from build123d import *

# Parameters (mm, degrees)
SKETCH2_R             = 0.5
BASE_DEPTH            = 2
M3_CLEARANCE_HOLE1_D  = 3.4
M4X0_7_TAPPED_HOLE1_D = 3.3


with BuildPart() as part:
    # Sketch2 → Base (new body, symmetric)
    with BuildSketch(Plane.XY):
        with BuildLine():
            Line((-18.5, 0), (18.5, 0))
            ThreePointArc((18.5, 0), (19.560660172, 0.439339828), (20, 1.5))
            Line((20, 1.5), (20, 1.8041591))
            ThreePointArc((20, 1.8041591), (20.327112072, 2.739217337), (21.165778543, 3.266450459))
            Line((21.165778543, 3.266450459), (46.691257218, 9.100556377))
            ThreePointArc((46.691257218, 9.100556377), (49.699443623, 13.891257218), (44.908742782, 16.899443623))
            Line((44.908742782, 16.899443623), (12.649834838, 9.526344449))
            ThreePointArc((12.649834838, 9.526344449), (10.989330142, 9.243827753), (9.307620269, 9.149258036))
            Line((9.307620269, 9.149258036), (-9.307620269, 9.149258036))
            ThreePointArc((-9.307620269, 9.149258036), (-10.989330142, 9.243827753), (-12.649834838, 9.526344449))
            Line((-12.649834838, 9.526344449), (-44.908742782, 16.899443623))
            ThreePointArc((-44.908742782, 16.899443623), (-49.699443623, 13.891257218), (-46.691257218, 9.100556377))
            Line((-46.691257218, 9.100556377), (-21.165778543, 3.266450459))
            ThreePointArc((-21.165778543, 3.266450459), (-20.327112072, 2.739217337), (-20, 1.8041591))
            Line((-20, 1.8041591), (-20, 1.5))
            ThreePointArc((-20, 1.5), (-19.560660172, 0.439339828), (-18.5, 0))
        make_face()
        with Locations((-45.8, 13)):
            Circle(SKETCH2_R, mode=Mode.SUBTRACT)
        with Locations((-8, 4)):
            Circle(SKETCH2_R, mode=Mode.SUBTRACT)
        with Locations((8, 4)):
            Circle(SKETCH2_R, mode=Mode.SUBTRACT)
        with Locations((45.8, 13)):
            Circle(SKETCH2_R, mode=Mode.SUBTRACT)
    extrude(amount=BASE_DEPTH, both=True)

    # M3 Clearance Hole1 (through all)
    with Locations(Plane(origin=(0, 4, 2), x_dir=(1, 0, 0), z_dir=(0, 0, 1))):
        with Locations((-8, 0), (8, 0)):
            Hole(M3_CLEARANCE_HOLE1_D / 2)

    # M4x0.7 Tapped Hole1 (through all)
    with Locations(Plane(origin=(0, 0, 2), x_dir=(-1, 0, 0), z_dir=(0, 0, 1))):
        with Locations((-45.8, -13), (45.8, -13)):
            Hole(M4X0_7_TAPPED_HOLE1_D / 2)


solid = part.part
Check sheet for the modelled part. Datum: model origin and axes. Units: mm. A direction names the side the tool comes from. Round coordinates to 2 decimals unless told otherwise and drop trailing zeros. Write each loop counter-clockwise with the first axis right and the second up, starting at its lowest first coordinate (ties: lowest second). Pieces come first, ordered by that corner, then holes. Notation, with made-up numbers: (-37, 67.25) - (-16, 67.25) arc R30 cw to (-16, 104.25) - close; hole circle Ø5 at (18, 69). An arc over 180 degrees is marked (long way). Return JSON: item names as keys, results as strings.
Q1. Draft check along Y on faces 1 (the cylindrical face through (-7.63, 2.34, -0.03)), 2 (the cylindrical face through (49.718, 13.805, 0.028)), 3 (the flat face through (-34.107, 6.224, 0.028)), 4 (the cylindrical face through (47.324, 13.632, -0.028)). Enter one of: released by +Y, released by -Y, zero draft, split by the parting line, or undercut.
Returned:
{"face 1": "undercut", "face 2": "split by the parting line", "face 3": "released by -Y", "face 4": "undercut"}
Q2. Cross-section at D-D (x = 42). Record the boundary of the cut face in (y, z).
Returned:
{"outline": "(8.03, -2) - (16.23, -2) - (16.23, 2) - (8.03, 2) - close"}
Q3. Scan lines: L1, parallel to Y at x = 8, z = 1.15; L2, parallel to X at y = 2.5, z = -1.25; L3, parallel to Y at x = -44.5, z = -1.75. Record each from-to range of solid material in increasing order. Write a range as from..to.
Returned:
{"L1": "y = 0..2.3, 5.7..9.15", "L2": "x = -20.17..-8.8, -7.2..7.2, 8.8..20.17", "L3": "y = 8.6..11.98, 14.02..16.81"}
Q4. Cross-section at A-A (x = -8). Record the boundary of the cut face in (y, z).
Returned:
{"outline": "(0, -2) - (2.3, -2) - (2.3, 2) - (0, 2) - close; (5.7, -2) - (9.15, -2) - (9.15, 2) - (5.7, 2) - close"}
Q5. Cross-section at C-C (z = 0). Record the boundary of the cut face in (x, y), then the cut area to 3 significant figures.
Returned:
{"outline": "(-46.69, 9.1) - (-21.17, 3.27) arc R1.5 cw to (-20, 1.8) - (-20, 1.5) arc R1.5 ccw to (-18.5, 0) - (18.5, 0) arc R1.5 ccw to (20, 1.5) - (20, 1.8) arc R1.5 cw to (21.17, 3.27) - (46.69, 9.1) arc R4 ccw to (44.91, 16.9) - (12.65, 9.53) arc R15 cw to (9.31, 9.15) - (-9.31, 9.15) arc R15 cw to (-12.65, 9.53) - (-44.91, 16.9) arc R4 ccw to start; hole circle Ø3.3 at (-45.8, 13); hole circle Ø3.4 at (-8, 4); hole circle Ø3.4 at (8, 4); hole circle Ø3.3 at (45.8, 13)", "area": "823 mm²"}
Q6. Cross-section at B-B (y = 15.5). Record the boundary of the cut face in (x, z).
Returned:
{"outline": "(-48.92, -2) - (-38.79, -2) - (-38.79, 2) - (-48.92, 2) - close; (38.79, -2) - (48.92, -2) - (48.92, 2) - (38.79, 2) - close"}
Q7. Depth check by flat-ended pin: P1, Ø3, axis at x = -8, y = 4, coming from the -Z side; P2, Ø1.2, axis at x = -2, z = 0.5, coming from the +Y side. Enter the tip coordinate at first touch or a pass-through.
Returned:
{"P1": "passes through", "P2": "stops at y = 9.15"}
Q8. Access from +Z, -Z, +X, -X, +Y, -Y to the whole of each face (thin tool, end or side, straight path). Record for faces 5 (the flat face through (-28.55, 13.16, 0.03)), 6 (the flat face through (-0.7, 8.6, 2)).
Returned:
{"face 5": "+Z, -Z, +Y", "face 6": "+Z, +X, -X, +Y, -Y"}
